Read the model definition and answer for the solid it produces. Units are mm, in the model's axes. Face numbers are marked on the shaded views. A direction names the side the tool comes from. Coordinates: 2 decimals unless noted, no trailing zeros. Loops run counter-clockwise (first coordinate to the right, second up) from the corner with the lowest first, then second, coordinate; pieces in that order, holes last.
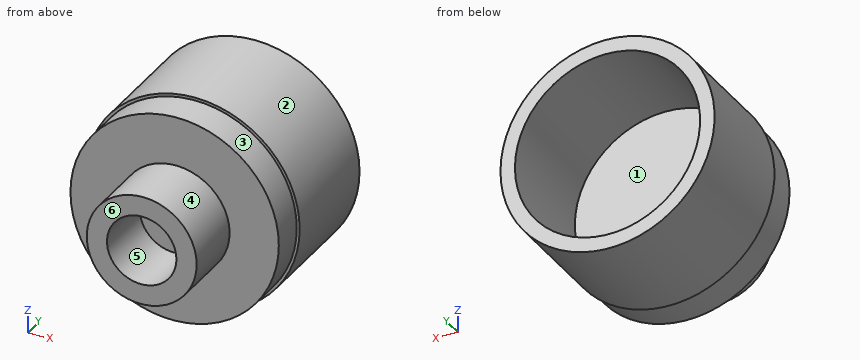
from build123d import *

# Parameters (mm, degrees)
F0_R     = 3.7
F0_R_2   = 3.2
F1_DEPTH = 4
F2_R     = 3.6
F3_DEPTH = 1.2
F4_R     = 1.9
F4_R_2   = 1.2
F5_DEPTH = 2.2


with BuildPart() as f1:
    # F0 (on Front) → F1 (new body)
    with BuildSketch(Plane.XZ):
        Circle(F0_R)
        Circle(F0_R_2, mode=Mode.SUBTRACT)
    extrude(amount=F1_DEPTH)

    # F2 (on face) → F3 (join)
    with BuildSketch(Plane.XZ.offset(4)):
        Circle(F2_R)
    extrude(amount=F3_DEPTH)

    # F4 (on face) → F5 (join)
    with BuildSketch(Plane.XZ.offset(5.2)):
        Circle(F4_R)
        Circle(F4_R_2, mode=Mode.SUBTRACT)
    extrude(amount=F5_DEPTH)


solid = f1.part
Q1. A cutting plane is placed at A-A (x = 0). Give the vertices of the cut face in (y, z), then the cut area to 3 significant figures.
Findings below:
outline: (-7.4, -1.9) - (-5.2, -1.9) - (-5.2, -3.6) - (-4, -3.6) - (-4, -3.7) - (0, -3.7) - (0, -3.2) - (-4, -3.2) - (-4, 3.2) - (0, 3.2) - (0, 3.7) - (-4, 3.7) - (-4, 3.6) - (-5.2, 3.6) - (-5.2, 1.9) - (-7.4, 1.9) - (-7.4, 1.2) - (-5.2, 1.2) - (-5.2, -1.2) - (-7.4, -1.2) - close
area: 15.7 mm2
Q2. A cutting plane is placed at D-D (y = -4.5). Give the vertices of the cut face in (x, z), then the cut area to 3 significant figures.
Findings below:
outline: circle Ø7.2 at (0, 0)
area: 40.7 mm2
Q3. A cutting plane is placed at C-C (y = -6.5). Give the vertices of the cut face in (x, z).
Findings below:
outline: circle Ø3.8 at (0, 0); hole circle Ø2.4 at (0, 0)
Q4. A cutting plane is placed at B-B (z = 0). Give the vertices of the cut face in (x, y), then the cut area to 3 significant figures.
Findings below:
outline: (-3.7, -4) - (-3.6, -4) - (-3.6, -5.2) - (-1.9, -5.2) - (-1.9, -7.4) - (-1.2, -7.4) - (-1.2, -5.2) - (1.2, -5.2) - (1.2, -7.4) - (1.9, -7.4) - (1.9, -5.2) - (3.6, -5.2) - (3.6, -4) - (3.7, -4) - (3.7, 0) - (3.2, 0) - (3.2, -4) - (-3.2, -4) - (-3.2, 0) - (-3.7, 0) - close
area: 15.7 mm2
Q5. Straight lines are drawn through the part: probe 1 along Z at (x, y) = (0, -2.4); probe 2 along Z at (x, y) = (0, -5.8); probe 3 along X at (y, z) = (-6, -0.25). For each, find the intervals that lie inside material, in ascending order.
Findings below:
probe 1: z = -3.7 to -3.2, 3.2 to 3.7
probe 2: z = -1.9 to -1.2, 1.2 to 1.9
probe 3: x = -1.88 to -1.17, 1.17 to 1.88
Q6. Which of the six approach directions +Z, -Z, +X, -X, +Y, -Y give full straight-line access (tool end or side, diameter ignored) to the marked faces 1, 2 and 3?
Findings below:
face 1: +Y
face 2: +Y, -Y
face 3: -Y
Q7. Flat-ended cylindrical pins translate along their axes: pin 1 Ø4 at (x, y) = (-1.5, -6) entering from -Z; pin 2 Ø4 at (y, z) = (-6, 2) entering from -X; pin 3 Ø1.5 at (x, y) = (2, -3) entering from +Z. Find the tip coordinate at first contact, or state that the pin passes through.
Findings below:
pin 1: stops at z = -3.6
pin 2: stops at x = -3.6
pin 3: stops at z = 3.48
Q8. Determine the mould class of the marked faces 4, 5 and 6 for opening direction X: +X half, -X half, draft (parallel to the pull), parting line (faces both ways), or undercut.
Findings below:
face 4: parting line
face 5: undercut
face 6: draft
